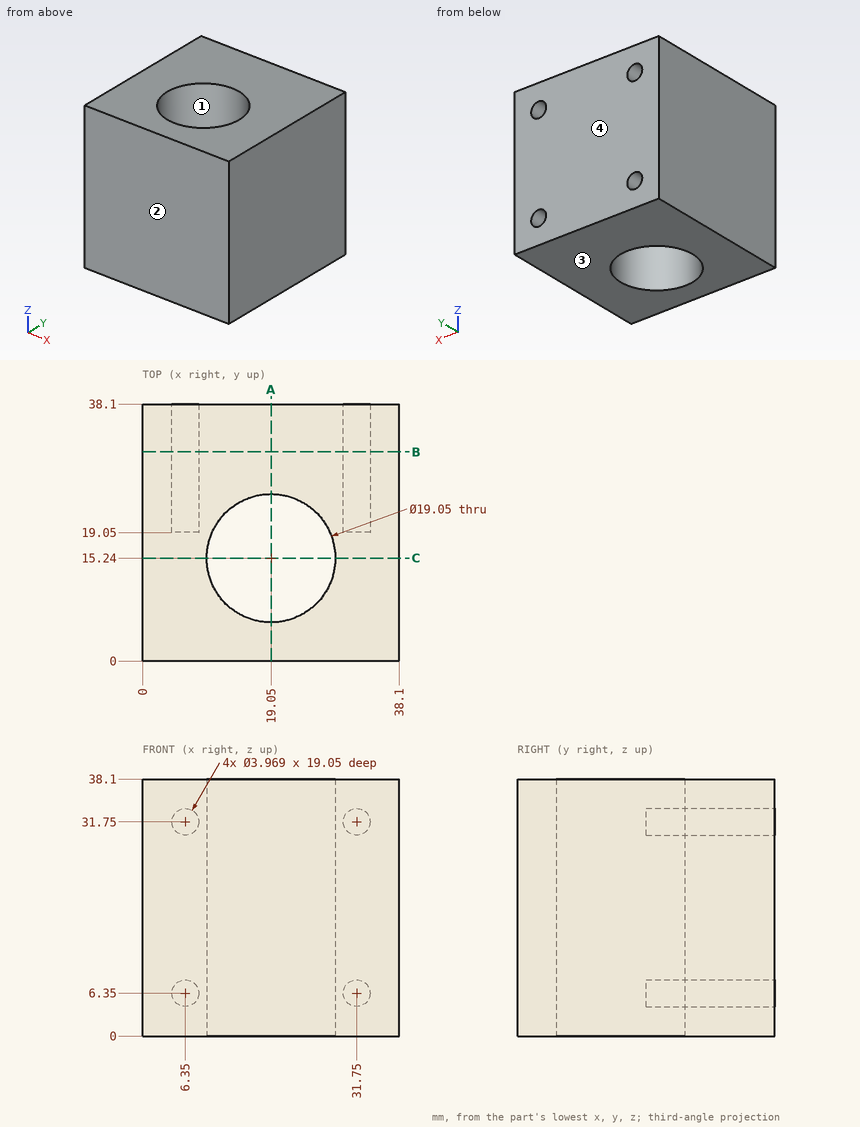
Input: dimensioned drawing with shaded views. Units: mm. Origin: part minimum x, y, z. Round coordinates to 2 decimals unless told otherwise and drop trailing zeros. Loops run counter-clockwise (first coordinate to the right, second up) from the corner with the lowest first, then second, coordinate; pieces in that order, holes last. Notation, with made-up numbers: M 32.5,-30 L 77.5,-30 A25 ccw 77.5,-18 Z; hole C 25.5,78.25 d6. An arc over 180 degrees is marked long. Answer in a Markdown table with one row per item. Add a question column.
1. Section B-B (y = 31). Output: boundary loops of the cut face in (x, z), and give its area (3 significant figures).
2. Ray query, probe 1 along X at (y, z) = (26.75, 31.75); probe 2 along X at (y, z) = (23, 6.35) (1 decimal). Return the intervals inside material, ascending.
3. Contact query for a flat-ended pin moving along its axis: pin 1 (2 mm diameter, centred on x = 31.5, z = 5.5, fed in from +Y). Output: stop coordinate, or through.
4. Section A-A (x = 19.05). Output: boundary loops of the cut face in (y, z) (1 decimal), and give its area (3 significant figures).
5. Section C-C (y = 15.24). Output: boundary loops of the cut face in (x, z) (1 decimal), and give its area (3 significant figures).
6. Mould query, pull axis Y, two halves, no side actions, for the marked faces 1, 2, 3 and 4. Classes: released by +Y, released by -Y, zero draft, split by the parting line, or undercut.
Values follow:
| question | item | result |
|---|---|---|
| 1 | outline | M 0,0 L 38.1,0 L 38.1,38.1 L 0,38.1 Z; hole C 6.35,6.35 d3.97; hole C 6.35,31.75 d3.97; hole C 31.75,6.35 d3.97; hole C 31.75,31.75 d3.97 |
| 1 | area | 1,400 mm^2 |
| 2 | probe 1 | 0 to 4.37, 8.33 to 29.77, 33.73 to 38.1 |
| 2 | probe 2 | 0 to 4.4, 8.3 to 13.5, 24.6 to 29.8, 33.7 to 38.1 |
| 3 | pin 1 | y = 19.05 |
| 4 | outline | M 0,0 L 5.7,0 L 5.7,38.1 L 0,38.1 Z; M 24.8,0 L 38.1,0 L 38.1,38.1 L 24.8,38.1 Z |
| 4 | area | 726 mm^2 |
| 5 | outline | M 0,0 L 9.5,0 L 9.5,38.1 L 0,38.1 Z; M 28.6,0 L 38.1,0 L 38.1,38.1 L 28.6,38.1 Z |
| 5 | area | 726 mm^2 |
| 6 | face 1 | undercut |
| 6 | face 2 | released by -Y |
| 6 | face 3 | zero draft |
| 6 | face 4 | released by +Y |
